from build123d import *

# Parameters (mm, degrees)
SKETCH1_R           = 13
BOSS_EXTRUDE1_DEPTH = 4
SKETCH2_R           = 7.25
CUT_EXTRUDE1_DEPTH  = 3
SKETCH3_R           = 1.5
CUT_EXTRUDE2_DEPTH  = 5
SKETCH6_R           = 6
BOSS_EXTRUDE5_DEPTH = 10
BOSS_EXTRUDE4_START = 10
SKETCH5_W           = 8
SKETCH5_H           = 8
BOSS_EXTRUDE4_DEPTH = 5
BOSS_EXTRUDE3_START = 15
SKETCH4_R           = 4
BOSS_EXTRUDE3_DEPTH = 30
SKETCH10_W          = 2
SKETCH10_H          = 1


with BuildPart() as part:
    # Sketch1 → Boss-Extrude1 (new body)
    with BuildSketch(Plane.XY):
        Circle(SKETCH1_R)
    extrude(amount=BOSS_EXTRUDE1_DEPTH)

    # Sketch2 → Cut-Extrude1 (cut)
    with BuildSketch(Plane(origin=(0, 0, 0), x_dir=(-1, 0, 0), z_dir=(0, 0, -1))):
        Circle(SKETCH2_R)
    extrude(amount=-CUT_EXTRUDE1_DEPTH, mode=Mode.SUBTRACT)

    # Sketch3 → Cut-Extrude2 (cut, through all)
    with BuildSketch(Plane.XY.offset(4)):
        with Locations((0, 10)):
            Circle(SKETCH3_R)
        with Locations((10, 0)):
            Circle(SKETCH3_R)
        with Locations((0, -10)):
            Circle(SKETCH3_R)
        with Locations((-10, 0)):
            Circle(SKETCH3_R)
    extrude(amount=-CUT_EXTRUDE2_DEPTH, mode=Mode.SUBTRACT)

    # Sketch6 → Boss-Extrude5 (add)
    with BuildSketch(Plane.XY.offset(4)):
        Circle(SKETCH6_R)
    extrude(amount=BOSS_EXTRUDE5_DEPTH)

    # Sketch5 → Boss-Extrude4 (add)
    with BuildSketch(Plane.XY.offset(4).offset(BOSS_EXTRUDE4_START)):
        Rectangle(SKETCH5_W, SKETCH5_H)
    extrude(amount=BOSS_EXTRUDE4_DEPTH)

    # Sketch4 → Boss-Extrude3 (add)
    with BuildSketch(Plane.XY.offset(4).offset(BOSS_EXTRUDE3_START)):
        Circle(SKETCH4_R)
    extrude(amount=BOSS_EXTRUDE3_DEPTH)

    # Sketch10 → Cut-Revolve1 (revolve, cut)
    with BuildSketch(Plane(origin=(0, 0, 0), x_dir=(1, 0, 0), z_dir=(0, 1, 0))):
        with Locations((-4.5, -39.5)):
            Rectangle(SKETCH10_W, SKETCH10_H)
    revolve(axis=Axis((0, 0, 0), (0, 0, 1)), mode=Mode.SUBTRACT)


solid = part.part
Input: part model. Units: mm. Frame: model coordinates. A direction names the side the tool comes from. Give positions to 0.01 mm unless a question says otherwise; leave off trailing zeros. Loops run counter-clockwise (first coordinate to the right, second up) from the corner with the lowest first, then second, coordinate; pieces in that order, holes last. Notation, with made-up numbers: (-37, 46.25) - (21, 46.25) arc R28 cw to (21, 70.25) - close; hole circle Ø4 at (-27.75, -12.75). An arc over 180 degrees is marked (long way). Use CSV: the item, a comma, the result in double quotes. Start each with the question number.
Item 1: Section C-C on y = 2.5. Return loops of the section in (x, z), then the cut area to 3 significant figures.
Item 2: Section D-D on z = 10. Return loops of the section in (x, y).
Item 3: Mould query, pull axis X, two halves, no side actions, for faces 6 (the flat face through (0, -4, 16)), 7 (the flat face through (0, 0, 3)), 8 (the flat face through (-4, 0, 16)), 9 (the cylindrical face through (-3.233, 1.341, 39.493)). Classes: pulls with the +X half, pulls with the -X half, needs draft (parallel to the pull), parting line crosses it, or undercut.
Item 4: Section A-A on x = -9.25. Return loops of the section in (y, z).
Item 5: Reachability of faces 1 (the flat face through (3, -3, 19)), 2 (the flat face through (4, 0, 16)), 3 (the flat face through (-3, -3, 19)), 4 (the flat face through (-4.5, 0.5, 14)), 5 (the flat face through (3, 3, 19)) from +Z, -Z, +X, -X, +Y, -Y: full face, straight path, thin tool, end or side. Return the list, or none.
Item 6: Line query: line 1 (Y direction, x = 0, z = 2.95); line 2 (Y direction, x = 0, z = 3.1); line 3 (Z direction, x = 0, y = -8). Output: solid intervals per line, ascending.
Item 7: Contact query for flat-ended pins moving along their axis: P1, Ø5.5, axis at x = -0.5, z = 17, coming from the -Y side; P2, Ø10, axis at y = -9.5, z = 20, coming from the +X side; P3, Ø8, axis at y = 3.5, z = 17.5, coming from the +X side; P4, Ø5, axis at x = -2.5, y = 2.5, coming from the -Z side. Output: stop coordinate, or through.
Item 8: Section B-B on y = -10. Return loops of the section in (x, z).
Ans:
1,outline,"(-12.76, 0) - (-6.81, 0) - (-6.81, 3) - (6.81, 3) - (6.81, 0) - (12.76, 0) - (12.76, 4) - (5.45, 4) - (5.45, 14) - (4, 14) - (4, 19) - (3.12, 19) - (3.12, 39) - (2.45, 39) - (2.45, 40) - (3.12, 40) - (3.12, 49) - (-3.12, 49) - (-3.12, 40) - (-2.45, 40) - (-2.45, 39) - (-3.12, 39) - (-3.12, 19) - (-4, 19) - (-4, 14) - (-5.45, 14) - (-5.45, 4) - (-12.76, 4) - close"
1,area,"396 mm2"
2,outline,"circle Ø12 at (0, 0)"
3,face 6,"needs draft"
3,face 7,"undercut"
3,face 8,"pulls with the -X half"
3,face 9,"parting line crosses it"
4,outline,"(-9.13, 0) - (-1.3, 0) - (-1.3, 4) - (-9.13, 4) - close; (1.3, 0) - (9.13, 0) - (9.13, 4) - (1.3, 4) - close"
5,face 1,"+Z, +X, -Y"
5,face 2,"+Z, +X, +Y, -Y"
5,face 3,"+Z, -X, -Y"
5,face 4,"+Z"
5,face 5,"+Z, +X, +Y"
6,line 1,"y = -13 to -11.5, -8.5 to -7.25, 7.25 to 8.5, 11.5 to 13"
6,line 2,"y = -13 to -11.5, -8.5 to 8.5, 11.5 to 13"
6,line 3,"z = 0 to 4"
7,P1,"stops at y = -4"
7,P2,"passes through"
7,P3,"stops at x = 5.79"
7,P4,"stops at z = 3"
8,outline,"(-8.31, 0) - (-1.5, 0) - (-1.5, 4) - (-8.31, 4) - close; (1.5, 0) - (8.31, 0) - (8.31, 4) - (1.5, 4) - close"
